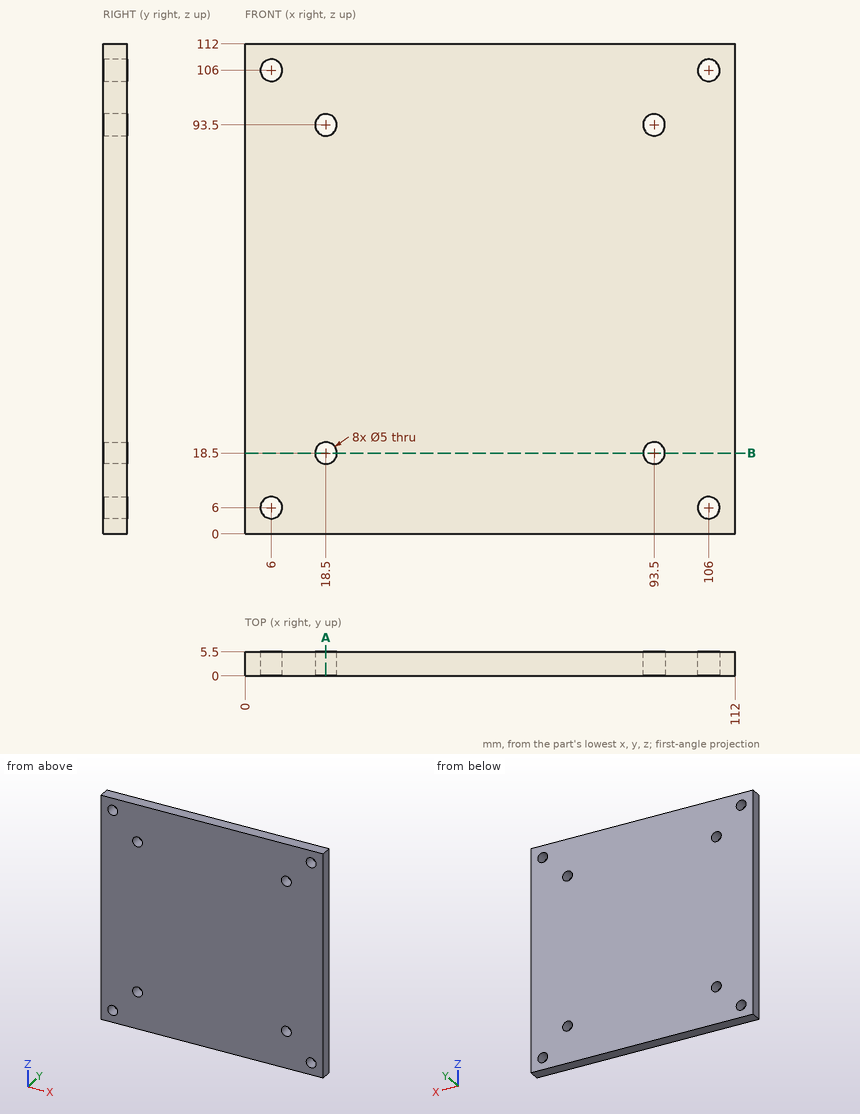
Verification items for this drawing (mm, ordinates from the low corner). Coordinates: 2 decimals unless noted, no trailing zeros. Order: outer loops, then holes, each group sorted by start corner. A loop starts at its lowest first (then second) coordinate and runs counter-clockwise, first axis right, second up. Notation, with made-up numbers: (89, -28.5) -> (120, -28.5) arc R34 cw to (120, 3.5) -> close; hole circle Ø1 at (21.25, -25.75). An arc over 180 degrees is marked (long way). Answer as CSV lines item,"result". Start each with the question number.
1) Material ranges on L1, parallel to Z at x = 6, y = 2.15; L2, parallel to Z at x = 18.5, y = 3.5, recorded low to high. Write a range as [from, to].
2) Cross-section at A-A, the plane x = 18.5. Record the boundary of the cut face in (y, z).
3) Cross-section at B-B, the plane z = 18.5. Record the boundary of the cut face in (x, y).
Conclusion:
1,L1,"z = [0, 3.5], [8.5, 103.5], [108.5, 112]"
1,L2,"z = [0, 16], [21, 91], [96, 112]"
2,outline,"(0, 0) -> (5.5, 0) -> (5.5, 16) -> (0, 16) -> close; (0, 21) -> (5.5, 21) -> (5.5, 91) -> (0, 91) -> close; (0, 96) -> (5.5, 96) -> (5.5, 112) -> (0, 112) -> close"
3,outline,"(0, 0) -> (16, 0) -> (16, 5.5) -> (0, 5.5) -> close; (21, 0) -> (91, 0) -> (91, 5.5) -> (21, 5.5) -> close; (96, 0) -> (112, 0) -> (112, 5.5) -> (96, 5.5) -> close"
